For this review, take the finished solid that the model builds, in its own axes (mm). A direction names the side the tool comes from. Give positions to 0.01 mm unless a question says otherwise; leave off trailing zeros. Loops run counter-clockwise (first coordinate to the right, second up) from the corner with the lowest first, then second, coordinate; pieces in that order, holes last. Notation, with made-up numbers: (20, -28.75) - (53, -28.75) arc R22 cw to (53, -8.75) - close; hole circle Ø7 at (52, 3). An arc over 180 degrees is marked (long way). Answer in a Markdown table with one row per item.
```python
from build123d import *

# Parameters (mm, degrees)
F0_W           = 19.05
F0_H           = 76.2
F1_DEPTH       = 12.7
F2_W           = 19.05
F2_H           = 12.7
F3_DEPTH       = 25.4
F5_D           = 6.35
F7_D           = 6.35
F7_CSINK_D     = 12.7
F7_CSINK_ANGLE = 90


with BuildPart() as f1:
    # F0 (on Front) → F1 (new body)
    with BuildSketch(Plane.XZ):
        Rectangle(F0_W, F0_H)
    extrude(amount=F1_DEPTH)

    # F2 (on face) → F3 (join)
    with BuildSketch(Plane.XZ.offset(12.7)):
        with Locations((0, -12.7)):
            Rectangle(F2_W, F2_H)
        with Locations((0, 12.7)):
            Rectangle(F2_W, F2_H)
    extrude(amount=F3_DEPTH)

    # F5 (through all)
    with Locations(Plane.XY.offset(19.05)):
        with Locations((0, -25.4)):
            Hole(F5_D / 2)

    # F7 (through all)
    with Locations(Plane.XZ.offset(12.7)):
        with Locations((0, 28.575), (0, -28.575)):
            CounterSinkHole(F7_D / 2, F7_CSINK_D / 2, counter_sink_angle=F7_CSINK_ANGLE)


solid = f1.part
```
1. Clearance check with flat-ended pins moving along their axes: pin 1 (1.5 mm diameter, centred on x = 0.5, z = 21.5, fed in from -Y); pin 2 (9.5 mm diameter, centred on x = -3, y = -31, fed in from +Z); pin 3 (7.5 mm diameter, centred on x = 0, z = 28.575, fed in from -Y). State where each tip first meets the part, or that it passes through.
Values:
| item | result |
|---|---|
| pin 1 | stops at y = -12.7 |
| pin 2 | stops at z = 19.05 |
| pin 3 | stops at y = -10.1 |
2. We need section B-B, the plane x = 0. Count the separate pieces of the cut face and the enclosed holes in it, and give its area (3 significant figures).
Values:
| item | result |
|---|---|
| separate pieces | 5 |
| enclosed holes | 0 |
| area | 1,270 mm^2 |
3. Wall thickness on line 1 (Z direction, x = 0, y = -3.75); line 2 (Y direction, x = 0, z = -10.5) (3 decimals); line 3 (Z direction, x = -8.5, y = -27): over which ranges is each line inside the solid? List them lowest first. Write a range as [from, to].
Values:
| item | result |
|---|---|
| line 1 | z = [-38.1, -31.75], [-25.4, 25.4], [31.75, 38.1] |
| line 2 | y = [-38.1, -28.575], [-22.225, 0] |
| line 3 | z = [-19.05, -6.35], [6.35, 19.05] |
4. We need section D-D, the plane y = -25.4. Give the boundary of the cut face in (x, z) (3 decimals).
Values:
| item | result |
|---|---|
| outline | (-9.525, -19.05) - (-3.175, -19.05) - (-3.175, -6.35) - (-9.525, -6.35) - close; (-9.525, 6.35) - (-3.175, 6.35) - (-3.175, 19.05) - (-9.525, 19.05) - close; (3.175, -19.05) - (9.525, -19.05) - (9.525, -6.35) - (3.175, -6.35) - close; (3.175, 6.35) - (9.525, 6.35) - (9.525, 19.05) - (3.175, 19.05) - close |
5. We need section C-C, the plane z = -16.5. Give the boundary of the cut face in (x, y) (3 decimals), and give its area (3 significant figures).
Values:
| item | result |
|---|---|
| outline | (-9.525, -38.1) - (9.525, -38.1) - (9.525, 0) - (-9.525, 0) - close; hole circle Ø6.35 at (0, -25.4) |
| area | 694 mm^2 |
6. For faces 4 (the face through (0.688, -4.696, 25.476)), 5 (the face through (-6.5, -12.7, -28.4)), 6 (the face through (0, -6, 38.1)), 7 (the face through (-2.3, -28, 19.05)), 8 (the face through (0, -12.7, 0)), list the 3-axis set-ups (+Z, -Z, +X, -X, +Y, -Y) from which the entire face can be reached by the end or side of a thin tool; tool diameter is ignored.
Values:
| item | result |
|---|---|
| face 4 | +Y, -Y |
| face 5 | -Z, +X, -X, -Y |
| face 6 | +Z, +X, -X, +Y, -Y |
| face 7 | +Z, +X, -X, -Y |
| face 8 | +X, -X, -Y |
7. Mouldability with a two-part tool opening along Z and no side actions: class faces 1 (the face through (9.525, -10, -1)), 2 (the face through (-2.3, -28, -19.05)), 3 (the face through (0.7, -9.7, 25.3)) as released by +Z, released by -Z, zero draft, split by the parting line, or undercut.
Values:
| item | result |
|---|---|
| face 1 | zero draft |
| face 2 | released by -Z |
| face 3 | undercut |
8. We need section A-A, the plane y = -20.5. Give the boundary of the cut face in (x, z) (3 decimals), and give its area (3 significant figures).
Values:
| item | result |
|---|---|
| outline | (-9.525, -19.05) - (9.525, -19.05) - (9.525, -6.35) - (-9.525, -6.35) - close; (-9.525, 6.35) - (9.525, 6.35) - (9.525, 19.05) - (-9.525, 19.05) - close |
| area | 484 mm^2 |
